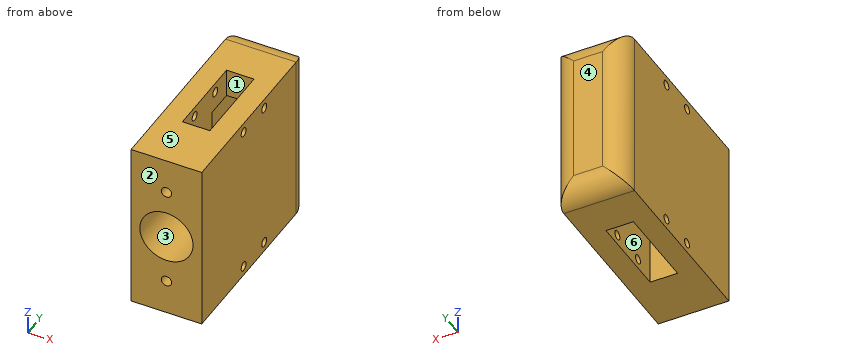
```python
from build123d import *

# Parameters (mm, degrees)
SKETCH1_W                    = 17
SKETCH1_H                    = 41
BOSS_EXTRUDE1_DEPTH          = 48
SKETCH2_W                    = 6.6
SKETCH2_H                    = 20.1
CUT_EXTRUDE1_DEPTH           = 64.696546217
SKETCH3_R                    = 1.105
CUT_EXTRUDE2_DEPTH           = 55.893077888
SKETCH4_R                    = 6.4
CUT_EXTRUDE3_DEPTH           = 42
FILLET3_R                    = 5
SKETCH8_W                    = 8
SKETCH8_H                    = 27.344585772
CUT_EXTRUDE4_DEPTH           = 15
TAP_DRILL_FOR_M3_TAP1_REACH  = 60.588
TAP_DRILL_FOR_M3_TAP1_BORE_R = 1.25


with BuildPart() as part:
    # Sketch1 → Boss-Extrude1 (new body)
    with BuildSketch(Plane(origin=(0, 0, 0), x_dir=(1, 0, 0), z_dir=(0, 1, 0))):
        Rectangle(SKETCH1_W, SKETCH1_H)
    extrude(amount=BOSS_EXTRUDE1_DEPTH)

    # Sketch2 → Cut-Extrude1 (cut, through all)
    with BuildSketch(Plane(origin=(0, 0, -20.5), x_dir=(-1, 0, 0), z_dir=(0, 0, -1))):
        with Locations((0, 23.582414356)):
            Rectangle(SKETCH2_W, SKETCH2_H)
    extrude(amount=-CUT_EXTRUDE1_DEPTH, mode=Mode.SUBTRACT)

    # Sketch3 → Cut-Extrude2 (cut, through all)
    with BuildSketch(Plane(origin=(8.5, 0, 0), x_dir=(0, 0, -1), z_dir=(1, 0, 0))):
        with Locations((-18.138, 19.075341505)):
            Circle(SKETCH3_R)
        with Locations((-18.138, 28.455341505)):
            Circle(SKETCH3_R)
        with Locations((18.138, 28.455341505)):
            Circle(SKETCH3_R)
        with Locations((18.138, 19.075341505)):
            Circle(SKETCH3_R)
    extrude(amount=-CUT_EXTRUDE2_DEPTH, mode=Mode.SUBTRACT)

    # Sketch4 → Cut-Extrude3 (cut)
    with BuildSketch(Plane.XZ):
        with Locations(Location((0, 0, 0), (0, 0, 270))):
            Circle(SKETCH4_R)
    extrude(amount=-CUT_EXTRUDE3_DEPTH, mode=Mode.SUBTRACT)

    # Fillet3
    fillet3_edges = [part.edges().sort_by_distance(p)[0] for p in [
        (-8.5, 48, 0),
        (0, 48, 20.5),
        (8.5, 48, 0),
        (0, 48, -20.5),
    ]]
    fillet(fillet3_edges, radius=FILLET3_R)

    # Sketch8 → Cut-Extrude4 (cut)
    with BuildSketch(Plane.XZ.offset(-42)):
        Rectangle(SKETCH8_W, SKETCH8_H)
    extrude(amount=CUT_EXTRUDE4_DEPTH, mode=Mode.SUBTRACT)

    # Tap Drill for M3 Tap1 bore (on position points) → Tap Drill for M3 Tap1 (cut, up to next)
    with BuildSketch(Plane(origin=(0, 0, -12), x_dir=(0, 0, -1), z_dir=(0, -1, 0)), mode=Mode.PRIVATE) as tap_drill_for_m3_tap1_sk1:
        Circle(TAP_DRILL_FOR_M3_TAP1_BORE_R)
    tap_drill_for_m3_tap1_tool1 = extrude(tap_drill_for_m3_tap1_sk1.sketch, amount=-TAP_DRILL_FOR_M3_TAP1_REACH, mode=Mode.PRIVATE) & part.part
    # Tap Drill for M3 Tap1 bore (on position points) → Tap Drill for M3 Tap1 (cut, up to next)
    with BuildSketch(Plane(origin=(0, 0, -12), x_dir=(0, 0, -1), z_dir=(0, -1, 0)), mode=Mode.PRIVATE) as tap_drill_for_m3_tap1_sk2:
        with Locations((-24, 0)):
            Circle(TAP_DRILL_FOR_M3_TAP1_BORE_R)
    tap_drill_for_m3_tap1_tool2 = extrude(tap_drill_for_m3_tap1_sk2.sketch, amount=-TAP_DRILL_FOR_M3_TAP1_REACH, mode=Mode.PRIVATE) & part.part
    add(tap_drill_for_m3_tap1_tool1.solids().sort_by_distance((0, 0, -12))[0], mode=Mode.SUBTRACT)
    add(tap_drill_for_m3_tap1_tool2.solids().sort_by_distance((0, 0, 12))[0], mode=Mode.SUBTRACT)


solid = part.part
```
Model file for the job. Use its own axes, mm. Face numbers are marked on the shaded views. A direction names the side the tool comes from. Round coordinates to 2 decimals unless told otherwise and drop trailing zeros. Write each loop counter-clockwise with the first axis right and the second up, starting at its lowest first coordinate (ties: lowest second). Pieces come first, ordered by that corner, then holes. Notation, with made-up numbers: (1.5, -0.75) - (43.5, -0.75) arc R33 ccw to (43.5, 36.25) - close; hole circle Ø1 at (49.25, -12.75). An arc over 180 degrees is marked (long way). Use CSV: the item, a comma, the result in double quotes. Start each with the question number.
Item 1: Drill centre lines: L1, parallel to Y at x = -2.25, z = -9.5; L2, parallel to Z at x = 3.5, y = 38.5; L3, parallel to X at y = 6.5, z = -12. Where is each one in solid material? Low to high. Write a range as [from, to].
Item 2: Band-saw the part on A-A (x = 0). Write the cut outline in (y, z), and give its area (3 significant figures).
Item 3: Band-saw the part on B-B (z = 8). Write the cut outline in (x, y).
Item 4: Tool access for the marked faces 5 and 6: list every direction of +Z, -Z, +X, -X, +Y, -Y with a clear straight run to the whole face (end or side of a thin tool).
Item 5: Band-saw the part on C-C (y = 38). Write the cut outline in (x, z), and give its area (3 significant figures).
Item 6: Two-plate mould, pull along Y, no slides. Class the marked faces 1, 2, 3 and 4: released by +Y, released by -Y, zero draft, split by the parting line, or undercut.
Item 7: Band-saw the part on D-D (y = 12). Write the cut outline in (x, z).
Item 8: Pin check, flat tips, straight feed: P1, Ø1, axis at x = -4, z = -9.5, coming from the -Y side; P2, Ø2, axis at x = 0, z = -12, coming from the -Y side. Stop position of each tip, or through.
Checked values:
1,L1,"y = [0, 13.53], [42, 48]"
1,L2,"z = [-20.5, -13.67], [13.67, 20.5]"
1,L3,"x = [-8.5, -1.25], [1.25, 8.5]"
2,outline,"(0, -20.5) - (13.53, -20.5) - (13.53, -13.25) - (0, -13.25) - close; (0, -10.75) - (13.53, -10.75) - (13.53, -6.4) - (0, -6.4) - close; (0, 6.4) - (13.53, 6.4) - (13.53, 10.75) - (0, 10.75) - close; (0, 13.25) - (13.53, 13.25) - (13.53, 20.5) - (0, 20.5) - close; (33.63, -20.5) - (43, -20.5) arc R5 ccw to (48, -15.5) - (48, 15.5) arc R5 ccw to (43, 20.5) - (33.63, 20.5) - (33.63, 13.67) - (42, 13.67) - (42, -13.67) - (33.63, -13.67) - close"
2,area,"663 mm²"
3,outline,"(-8.5, 0) - (8.5, 0) - (8.5, 43) arc R5 ccw to (3.5, 48) - (-3.5, 48) arc R5 ccw to (-8.5, 43) - close; hole (-4, 27) - (-3.3, 27) - (-3.3, 13.53) - (3.3, 13.53) - (3.3, 27) - (4, 27) - (4, 42) - (-4, 42) - close"
4,face 5,"+Z, +X, -X, +Y, -Y"
4,face 6,"+Z, -Z"
5,outline,"(-8.5, -20.5) - (8.5, -20.5) - (8.5, 20.5) - (-8.5, 20.5) - close; hole (-4, -13.67) - (4, -13.67) - (4, -5) arc R6.4 ccw to (4, 5) - (4, 13.67) - (-4, 13.67) - (-4, 5) arc R6.4 ccw to (-4, -5) - close"
5,area,"445 mm²"
6,face 1,"undercut"
6,face 2,"released by -Y"
6,face 3,"zero draft"
6,face 4,"released by +Y"
7,outline,"(-8.5, -20.5) - (8.5, -20.5) - (8.5, 20.5) - (-8.5, 20.5) - close; hole circle Ø12.8 at (0, 0); hole circle Ø2.5 at (0, -12); hole circle Ø2.5 at (0, 12)"
8,P1,"stops at y = 0"
8,P2,"stops at y = 42"
